Design review of the part built by this model. Coordinates are the model's own, in mm. Face numbers are marked on the shaded views. A direction names the side the tool comes from. Coordinates: 2 decimals unless noted, no trailing zeros. Loops run counter-clockwise (first coordinate to the right, second up) from the corner with the lowest first, then second, coordinate; pieces in that order, holes last. Notation, with made-up numbers: (-15.5, 78) -> (27.5, 78) arc R20 cw to (27.5, 87) -> close; hole circle Ø3 at (18.5, -29). An arc over 180 degrees is marked (long way). Use a Markdown table: item, result. Add a question column.
Q1. Take a section at A-A on x = 0. Count the separate pieces of the cut face and the enclosed holes in it, plus the area to 3 significant figures.
Q2. Draft analysis for pull direction X (two halves, no side actions). For the marked faces 1, 2, 3 and 4, state which applies: pulls with the +X half, pulls with the -X half, needs draft (parallel to the pull), parting line crosses it, or undercut.
Q3. Clearance check with flat-ended pins moving along their axes: pin 1 Ø4 at (y, z) = (13, -1.5) entering from -X; pin 2 Ø5 at (x, y) = (-6, 3.5) entering from +Z; pin 3 Ø12 at (y, z) = (8, -13) entering from +X; pin 4 Ø2 at (x, z) = (14, 0) entering from +Y. State where each tip first meets the part, or that it passes through.
Q4. Take a section at D-D on y = 18. Write out the cut boundary in (x, z), plus the area to 3 significant figures.
Q5. Take a section at C-C on y = 12.5. Write out the cut boundary in (x, z), plus the area to 3 significant figures.
Q6. Take a section at B-B on x = 14. Write out the cut boundary in (y, z).
Q7. For probe 1 along X at (y, z) = (0.4, 0); probe 2 along X at (y, z) = (2.5, 2); probe 3 along Y at (x, z) = (-10.5, -4.5), list the stretches that pass through material, from the lowest coordinate up.
Q8. For the marked faces 5 and 6, list the 3-axis set-ups (+Z, -Z, +X, -X, +Y, -Y) from which the entire face can be reached by the end or side of a thin tool; tool diameter is ignored.
from build123d import *

# Parameters (mm, degrees)
SKETCH1_R               = 17.5
BOSS_EXTRUDE1_DEPTH     = 3
SKETCH2_R               = 7
BOSS_EXTRUDE2_DEPTH     = 12.75
SKETCH3_R               = 7
SKETCH3_R_2             = 4.5
BOSS_EXTRUDE3_DEPTH     = 4.8
SKETCH4_R               = 2.5
CUT_EXTRUDE1_DEPTH      = 19.8
FILLET1_R               = 5
SKETCH5_R               = 1.25
CUT_EXTRUDE2_DEPTH      = 3
CUT_EXTRUDE3_DEPTH      = 1.5
CUT_EXTRUDE3_DEPTH_BACK = 1.5


with BuildPart() as part:
    # Sketch1 → Boss-Extrude1 (new body)
    with BuildSketch(Plane(origin=(0, 0, 0), x_dir=(1, 0, 0), z_dir=(0, 1, 0))):
        with Locations(Location((0, 0, 0), (0, 0, 270))):
            Circle(SKETCH1_R)
    extrude(amount=BOSS_EXTRUDE1_DEPTH)

    # Sketch2 → Boss-Extrude2 (add)
    with BuildSketch(Plane(origin=(0, 3, 0), x_dir=(1, 0, 0), z_dir=(0, 1, 0))):
        with Locations(Location((0, 0, 0), (0, 0, 270))):
            Circle(SKETCH2_R)
    extrude(amount=BOSS_EXTRUDE2_DEPTH)

    # Sketch3 → Boss-Extrude3 (add)
    with BuildSketch(Plane(origin=(0, 15.75, 0), x_dir=(1, 0, 0), z_dir=(0, 1, 0))):
        with Locations(Location((0, 0, 0), (0, 0, 270))):
            Circle(SKETCH3_R)
        with Locations(Location((0, 0, 0), (0, 0, 270))):
            Circle(SKETCH3_R_2, mode=Mode.SUBTRACT)
    extrude(amount=BOSS_EXTRUDE3_DEPTH)

    # Sketch4 → Cut-Extrude1 (cut)
    with BuildSketch(Plane(origin=(0, 15.75, 0), x_dir=(1, 0, 0), z_dir=(0, 1, 0))):
        with Locations(Location((0, 0, 0), (0, 0, 270))):
            Circle(SKETCH4_R)
    extrude(amount=-CUT_EXTRUDE1_DEPTH, mode=Mode.SUBTRACT)

    # Fillet1
    fillet1_edges = [part.edges().sort_by_distance(p)[0] for p in [
        (0, 3, -7),
    ]]
    fillet(fillet1_edges, radius=FILLET1_R)

    # Sketch5 → Cut-Extrude2 (cut)
    with BuildSketch(Plane(origin=(0, 3, 0), x_dir=(1, 0, 0), z_dir=(0, 1, 0))):
        with Locations(Location((0, 14, 0), (0, 0, 270))):
            Circle(SKETCH5_R)
        with Locations(Location((14, 0, 0), (0, 0, 270))):
            Circle(SKETCH5_R)
        with Locations(Location((0, -14, 0), (0, 0, 270))):
            Circle(SKETCH5_R)
        with Locations(Location((-14, 0, 0), (0, 0, 270))):
            Circle(SKETCH5_R)
    extrude(amount=-CUT_EXTRUDE2_DEPTH, mode=Mode.SUBTRACT)

    # Sketch6 → Cut-Extrude3 (cut, two sides: drawn at the far end of the back side and taken through both)
    with BuildSketch(Plane(origin=(0, 3, 0), x_dir=(1, 0, 0), z_dir=(0, 1, 0)).offset(-CUT_EXTRUDE3_DEPTH_BACK)):
        Polygon((2.886751346, 14), (1.443375673, 16.5), (-1.443375673, 16.5), (-2.886751346, 14), (-1.443375673, 11.5), (1.443375673, 11.5), align=None)
        Polygon((16.886751346, 0), (15.443375673, 2.5), (12.556624327, 2.5), (11.113248654, 0), (12.556624327, -2.5), (15.443375673, -2.5), align=None)
        Polygon((2.886751346, -14), (1.443375673, -11.5), (-1.443375673, -11.5), (-2.886751346, -14), (-1.443375673, -16.5), (1.443375673, -16.5), align=None)
        Polygon((-11.113248654, 0), (-12.556624327, 2.5), (-15.443375673, 2.5), (-16.886751346, 0), (-15.443375673, -2.5), (-12.556624327, -2.5), align=None)
    extrude(amount=CUT_EXTRUDE3_DEPTH + CUT_EXTRUDE3_DEPTH_BACK, mode=Mode.SUBTRACT)


solid = part.part
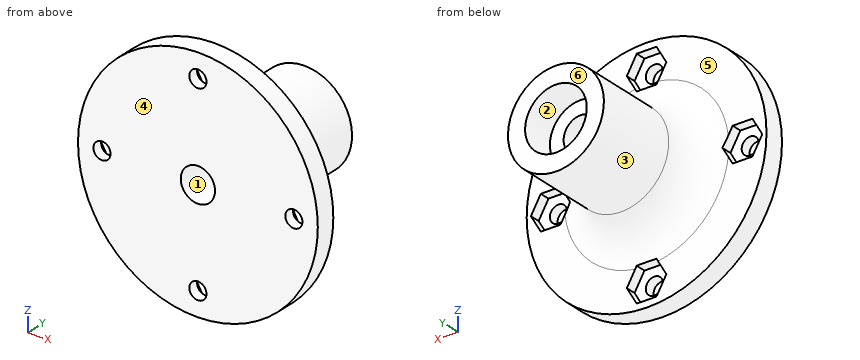
Answer list:
| question | item | result |
|---|---|---|
| 1 | separate pieces | 4 |
| 1 | enclosed holes | 0 |
| 1 | area | 217 mm² |
| 2 | face 1 | undercut |
| 2 | face 2 | undercut |
| 2 | face 3 | parting line crosses it |
| 2 | face 4 | needs draft |
| 3 | pin 1 | x = -7 |
| 3 | pin 2 | z = 17.14 |
| 3 | pin 3 | x = 14.58 |
| 3 | pin 4 | through |
| 4 | outline | circle Ø14 at (0, 0); hole circle Ø9 at (0, 0) |
| 4 | area | 90.3 mm² |
| 5 | outline | circle Ø14 at (0, 0); hole circle Ø5 at (0, 0) |
| 5 | area | 134 mm² |
| 6 | outline | (0, -10.5) -> (3, -10.5) -> (3, -2.5) -> (1.5, -2.5) -> (1.5, -1.25) -> (0, -1.25) -> close; (0, 1.25) -> (1.5, 1.25) -> (1.5, 2.5) -> (3, 2.5) -> (3, 10.5) -> (0, 10.5) -> close |
| 7 | probe 1 | -17.5 to -15.25, -12.75 to -2.5, 2.5 to 12.75, 15.25 to 17.5 |
| 7 | probe 2 | -17.39 to -15.73, -12.27 to -1.5, 1.5 to 12.27, 15.73 to 17.39 |
| 7 | probe 3 | 0 to 3.03 |
| 8 | face 5 | +Y |
| 8 | face 6 | +Z, -Z, +X, -X, +Y |
